from build123d import *

# Parameters (mm, degrees)
F0_W        = 7.62
F0_H        = 5.08
F0_W_2      = 12.7
F0_W_3      = 1.27
F0_H_2      = 4.6902727336
F0_H_3      = 2.9297272664
F0_W_4      = 101.6
F1_DEPTH    = 12.7
F2_T1_DEPTH = 19.05
F3_R        = 1.524
F4_DEPTH    = 25.4
F5_R        = 2.54


# Not quite as in the source:
# - a fillet or chamfer that OpenCascade refuses, or shapes differently, is made with other operations: its cross-section is extruded or revolved along the edge and cut away or added


with BuildPart() as f1:
    # F0 (on Top) → F1 (new body)
    with BuildSketch(Plane.XY):
        Polygon((-47.2217758975, 22.7881683916), (-54.8417758975, 22.7881683916), (-54.8417758975, -14.4997123967), (-47.2217758975, -14.4997123967), (-47.2217758975, 10.9002876033), (-47.2217758975, 13.8300148697), (-47.2217758975, 18.5202876033), (-51.7937758975, 18.5202876033), (-51.7937758975, 20.344916165), (-47.2217758975, 20.344916165), align=None)
        with Locations((-51.0317758975, -17.0397123967)):
            Rectangle(F0_W, F0_H)
        with Locations((-61.1917758975, -17.0397123967)):
            Rectangle(F0_W_2, F0_H)
        Polygon((64.5382241025, 22.7881683916), (56.9182241025, 22.7881683916), (56.9182241025, 20.344916165), (61.4902241025, 20.344916165), (61.4902241025, 18.5202876033), (56.9182241025, 18.5202876033), (56.9182241025, 13.8300148697), (56.9182241025, 10.9002876033), (56.9182241025, -14.4997123967), (64.5382241025, -14.4997123967), align=None)
        with Locations((-46.5867758975, 16.1751512365)):
            Rectangle(F0_W_3, F0_H_2)
        with Locations((60.7282241025, -17.0397123967)):
            Rectangle(F0_W, F0_H)
        with Locations((-46.5867758975, 12.3651512365)):
            Rectangle(F0_W_3, F0_H_3)
        with Locations((70.8882241025, -17.0397123967)):
            Rectangle(F0_W_2, F0_H)
        with Locations((56.2832241025, 16.1751512365)):
            Rectangle(F0_W_3, F0_H_2)
        with Locations((56.2832241025, 12.3651512365)):
            Rectangle(F0_W_3, F0_H_3)
        with Locations((4.8482241025, 12.3651512365)):
            Rectangle(F0_W_4, F0_H_3)
    extrude(amount=F1_DEPTH)

    # F2: fillet of radius 1.27 on 6 edges, made by hand

    # F2_s2 → F2_t1 (cut)
    with BuildSketch(Plane.XY.offset(-3.175)):
        with BuildLine():
            ThreePointArc((-48.4917758975, 22.7881683916), (-47.5937502854, 22.4161940037), (-47.2217758975, 21.5181683916))
            Line((-47.2217758975, 21.5181683916), (-47.2217758975, 22.7881683916))
            Line((-47.2217758975, 22.7881683916), (-48.4917758975, 22.7881683916))
        make_face()
        with BuildLine():
            ThreePointArc((-45.9517758975, 17.2502876033), (-46.3237502854, 18.1483132154), (-47.2217758975, 18.5202876033))
            Line((-47.2217758975, 18.5202876033), (-45.9517758975, 18.5202876033))
            Line((-45.9517758975, 18.5202876033), (-45.9517758975, 17.2502876033))
        make_face()
        with BuildLine():
            ThreePointArc((-48.4917758975, 20.344916165), (-47.5937502854, 20.7168905529), (-47.2217758975, 21.614916165))
            Line((-47.2217758975, 21.614916165), (-47.2217758975, 20.344916165))
            Line((-47.2217758975, 20.344916165), (-48.4917758975, 20.344916165))
        make_face()
        with BuildLine():
            ThreePointArc((56.9182241025, 18.5202876033), (56.0201984904, 18.1483132154), (55.6482241025, 17.2502876033))
            Line((55.6482241025, 17.2502876033), (55.6482241025, 18.5202876033))
            Line((55.6482241025, 18.5202876033), (56.9182241025, 18.5202876033))
        make_face()
        with BuildLine():
            ThreePointArc((56.9182241025, 21.614916165), (57.2901984904, 20.7168905529), (58.1882241025, 20.344916165))
            Line((58.1882241025, 20.344916165), (56.9182241025, 20.344916165))
            Line((56.9182241025, 20.344916165), (56.9182241025, 21.614916165))
        make_face()
        with BuildLine():
            ThreePointArc((58.1882241025, 22.7881683916), (57.2901984904, 22.4161940037), (56.9182241025, 21.5181683916))
            Line((56.9182241025, 21.5181683916), (56.9182241025, 22.7881683916))
            Line((56.9182241025, 22.7881683916), (58.1882241025, 22.7881683916))
        make_face()
    extrude(amount=F2_T1_DEPTH, mode=Mode.SUBTRACT)

    # F3 (on face) → F4 (cut)
    with BuildSketch(Plane.XZ.offset(19.5797123967)):
        with Locations((-61.1917758975, 6.35)):
            Circle(F3_R)
        with Locations((70.8882241025, 6.35)):
            Circle(F3_R)
    extrude(amount=-F4_DEPTH, mode=Mode.SUBTRACT)

    # F5
    f5_edges = [f1.edges().sort_by_distance(p)[0] for p in [
        (77.238224, -17.039712, 12.7),
        (77.238224, -17.039712, 0),
        (64.538224, 22.788168, 6.35),
        (-54.841776, 22.788168, 6.35),
        (-67.541776, -17.039712, 0),
        (-67.541776, -17.039712, 12.7),
        (-54.841776, 4.144228, 0),
        (-54.841776, 4.144228, 12.7),
        (64.538224, 4.144228, 0),
        (64.538224, 4.144228, 12.7),
    ]]
    fillet(f5_edges, radius=F5_R)


solid = f1.part
Check sheet for the modelled part. Datum: model origin and axes. Units: mm. A direction names the side the tool comes from. Give positions to 0.01 mm unless a question says otherwise; leave off trailing zeros. Write each loop counter-clockwise with the first axis right and the second up, starting at its lowest first coordinate (ties: lowest second). Pieces come first, ordered by that corner, then holes. Notation, with made-up numbers: (-16, 38) -> (-3, 38) arc R12 cw to (-3, 42) -> close; hole circle Ø1 at (4.5, 45). An arc over 180 degrees is marked (long way). One line per item, written item: value. Start each with the question number.
Item 1: Tool access check on faces 5 (the flat face through (64.538, 3, 6)), 6 (the cylindrical face through (-54.078, 3.883, 0.724)), 7 (the flat face through (-45.952, 16, 6)). Record the directions out of +Z, -Z, +X, -X, +Y, -Y that give a thin tool (end or side, any length) a straight path to the whole face; none if there is none.
Item 2: Material ranges on probe 1 along X at (y, z) = (14.5, 2.75); probe 2 along X at (y, z) = (-8.5, 3.75); probe 3 along Y at (x, z) = (51, 10.5), recorded low to high. Write a range as from..to.
Item 3: Section check A-A on y = -16.5. Record the cut outline in (x, z), then the cut area to 3 significant figures.
Item 4: Gauge pin test, flat ends, axial feed: pin 1 (4 mm diameter, centred on x = 30, y = 16, fed in from -Z); pin 2 (2.5 mm diameter, centred on y = 15, z = 4, fed in from -X); pin 3 (2 mm diameter, centred on x = 33, z = 4, fed in from -Y); pin 4 (1 mm diameter, centred on x = -27.5, z = 10, fed in from +Y). Record the tip position at first contact, or that the pin passes through.
Item 5: Section check C-C on z = 6.35. State how many separate pieces and enclosed holes the cut face has, then the cut area to 3 significant figures.
Item 6: Section check D-D on x = 49. Record the cut outline in (y, z).
Item 7: Section check B-B on y = -3. Record the cut outline in (x, z).
Item 8: Draft check along X on faces 1 (the cylindrical face through (-59.74, -17.08, 6.81)), 2 (the cylindrical face through (63.77, 4.41, 0.72)), 3 (the flat face through (67, -19.58, 6)), 4 (the flat face through (4, 13.83, 6)). Enter one of: +X half, -X half, draft (parallel to the pull), parting line (faces both ways), or undercut.
Results list:
1. face 5: +Z, -Z, +X, +Y
1. face 6: -Z, -X, +Y
1. face 7: +Z, -Z, +Y
2. probe 1: -54.84..-45.95, 55.65..64.54
2. probe 2: -54.84..-47.22, 56.92..64.54
2. probe 3: 10.9..13.83
3. outline: (-67.54, 2.54) arc R2.54 ccw to (-65, 0) -> (-47.22, 0) -> (-47.22, 12.7) -> (-65, 12.7) arc R2.54 ccw to (-67.54, 10.16) -> close; (56.92, 0) -> (74.7, 0) arc R2.54 ccw to (77.24, 2.54) -> (77.24, 10.16) arc R2.54 ccw to (74.7, 12.7) -> (56.92, 12.7) -> close; hole circle Ø3.05 at (-61.19, 6.35); hole circle Ø3.05 at (70.89, 6.35)
3. area: 496 mm²
4. pin 1: through
4. pin 2: x = -54.84
4. pin 3: y = 10.9
4. pin 4: y = 13.83
5. separate pieces: 3
5. enclosed holes: 0
5. area: 1,040 mm²
6. outline: (10.9, 0) -> (13.83, 0) -> (13.83, 12.7) -> (10.9, 12.7) -> close
7. outline: (-54.84, 2.54) arc R2.54 ccw to (-52.3, 0) -> (-47.22, 0) -> (-47.22, 12.7) -> (-52.3, 12.7) arc R2.54 ccw to (-54.84, 10.16) -> close; (56.92, 0) -> (62, 0) arc R2.54 ccw to (64.54, 2.54) -> (64.54, 10.16) arc R2.54 ccw to (62, 12.7) -> (56.92, 12.7) -> close
8. face 1: undercut
8. face 2: +X half
8. face 3: draft
8. face 4: undercut
